Check sheet for the modelled part. Datum: model origin and axes. Units: mm. A direction names the side the tool comes from. Give positions to 0.01 mm unless a question says otherwise; leave off trailing zeros. Order: outer loops, then holes, each group sorted by start corner. A loop starts at its lowest first (then second) coordinate and runs counter-clockwise, first axis right, second up.
```python
from build123d import *

# Parameters (mm, degrees)
FILLET1_R = 0.15
FILLET2_R = 0.15


with BuildPart() as part:
    # Sketch1 → Revolve1 (revolve)
    with BuildSketch(Plane.XY):
        Polygon((0, 2.5), (5, 2.5), (5, 3.46), (4.88, 3.46), (4.88, 4.7675), (5, 4.7675), (5, 5.5), (0, 5.5), (0, 4.7675), (0.12, 4.7675), (0.12, 3.46), (0, 3.46), align=None)
    revolve(axis=Axis((0, 0, 0), (1, 0, 0)))

    # Fillet1
    fillet1_edges = [part.edges().sort_by_distance(p)[0] for p in [
        (0, -5.5, 0),
        (5, -5.5, 0),
    ]]
    fillet(fillet1_edges, radius=FILLET1_R)

    # Fillet2
    fillet2_edges = [part.edges().sort_by_distance(p)[0] for p in [
        (5, -2.5, 0),
        (0, -2.5, 0),
    ]]
    fillet(fillet2_edges, radius=FILLET2_R)


solid = part.part
```
(1) Tool access check on faces 4 (the face through (4.88, 0, 4)), 5 (the face through (5, 4, -3)), 6 (the face through (0.12, 0, 4)). Record the directions out of +Z, -Z, +X, -X, +Y, -Y that give a thin tool (end or side, any length) a straight path to the whole face; none if there is none.
(2) Release check for a two-part mould opening along Z. For faces 1 (the face through (2.47, -1.19, -5.37)), 2 (the face through (2.53, -0.54, -2.44)), 3 (the face through (0, -4, -3)) record: released by +Z, released by -Z, zero draft, split by the parting line, or undercut.
(3) Go/stop test with flat-tipped pins: P1, Ø1.5, axis at x = 2.5, z = 2, coming from the +Y side; P2, Ø1, axis at x = 4.5, z = -3.5, coming from the -Y side; P3, Ø3, axis at y = 0, z = 0, coming from the +X side. Record where each tip stops, or that it passes through.
(4) Thickness scan on L1, parallel to Z at x = 1.4, y = 0; L2, parallel to Z at x = 4.95, y = 0; L3, parallel to X at y = -3, z = 3.25. Record the ranges inside material, lowest first.
(5) Sectioned sample at C-C (x = 3.4). Enter the section's corners in (y, z), plus the area to 3 significant figures.
Values follow:
1. face 4: +X
1. face 5: +Z, -Z, +X, +Y, -Y
1. face 6: -X
2. face 1: split by the parting line
2. face 2: undercut
2. face 3: zero draft
3. P1: stops at y = 5.36
3. P2: stops at y = -4.61
3. P3: passes through
4. L1: z = -5.5 to -2.5, 2.5 to 5.5
4. L2: z = -5.46 to -4.77, -3.46 to -2.54, 2.54 to 3.46, 4.77 to 5.46
4. L3: x = 0.12 to 4.88
5. outline: circle Ø11 at (0, 0); hole circle Ø5 at (0, 0)
5. area: 75.4 mm2
